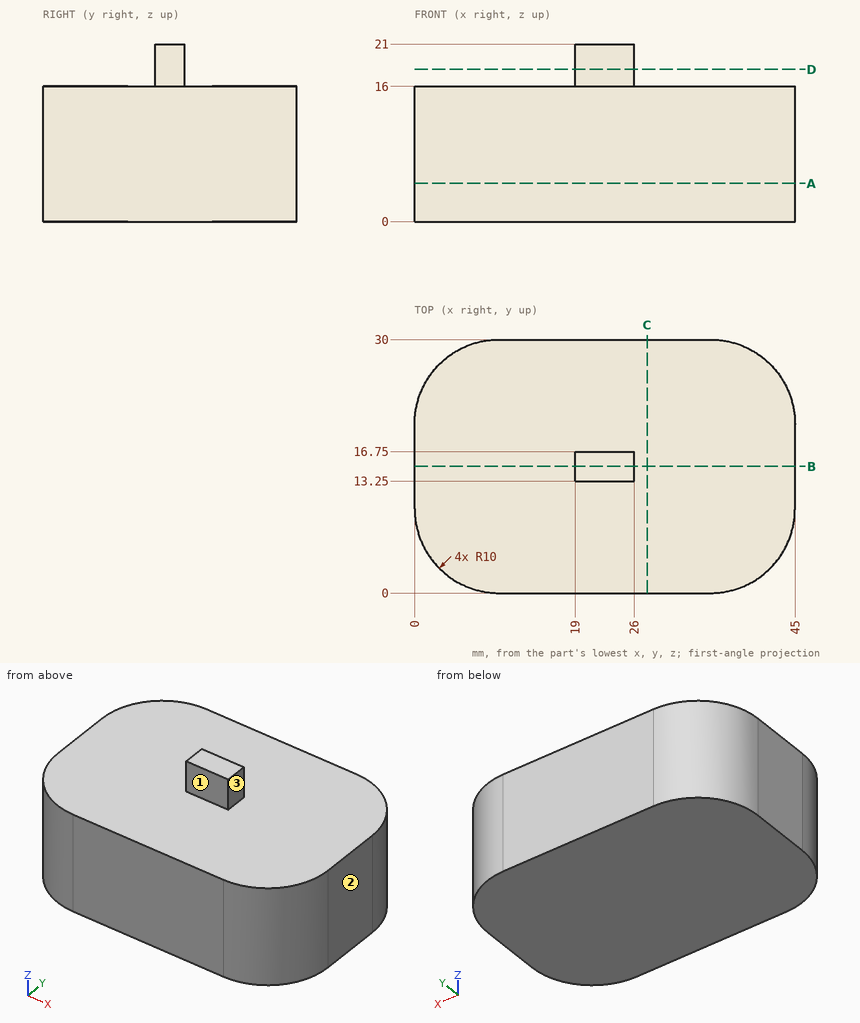
Here's the drawing with two shaded views (mm, measured from the low corner). I have some questions. A direction names the side the tool comes from. Coordinates: 2 decimals unless noted, no trailing zeros. Write each loop counter-clockwise with the first axis right and the second up, starting at its lowest first coordinate (ties: lowest second). Pieces come first, ordered by that corner, then holes. Notation, with made-up numbers: M -34.75,69 L 23.25,69 A22 cw 23.25,93 Z; hole C 14.25,-36.75 d9. An arc over 180 degrees is marked long. Answer as CSV lines item,"result".
Item 1: Imagine slicing it at B-B on y = 15. List the corners of the cut face in (x, z) for me, plus the area to 3 significant figures.
Geometry results:
outline,"M 0,0 L 45,0 L 45,16 L 26,16 L 26,21 L 19,21 L 19,16 L 0,16 Z"
area,"755 mm2"
Item 2: Imagine slicing it at A-A on z = 4.5. List the corners of the cut face in (x, y) for me.
Geometry results:
outline,"M 0,10 A10 ccw 10,0 L 35,0 A10 ccw 45,10 L 45,20 A10 ccw 35,30 L 10,30 A10 ccw 0,20 Z"
Item 3: I'm going to push flat-ended pins straight in: P1, Ø3, axis at y = 27, z = 9, coming from the +X side; P2, Ø1.5, axis at x = 24, z = 19.5, coming from the -Y side; P3, Ø2, axis at x = 7.5, y = 15, coming from the +Z side; P4, Ø6, axis at y = 7, z = 3, coming from the +X side. Where does each tip first touch, or does it pass through?
Geometry results:
P1,"stops at x = 43.35"
P2,"stops at y = 13.25"
P3,"stops at z = 16"
P4,"stops at x = 45"
Item 4: On a 3-axis mill with a long thin cutter (end or side, diameter ignored), from which of +Z, -Z, +X, -X, +Y, -Y can I reach the whole of each face in a straight line? I mean the marked faces 1, 2 and 3. Say none if no direction works.
Geometry results:
face 1,"+Z, +X, -X, -Y"
face 2,"+Z, -Z, +X, +Y, -Y"
face 3,"+Z, +X, +Y, -Y"
Item 5: Imagine slicing it at D-D on z = 18. List the corners of the cut face in (x, y) for me, plus the area to 3 significant figures.
Geometry results:
outline,"M 19,13.25 L 26,13.25 L 26,16.75 L 19,16.75 Z"
area,"24.5 mm2"
Item 6: Imagine slicing it at C-C on x = 27.5. List the corners of the cut face in (y, z) for me.
Geometry results:
outline,"M 0,0 L 30,0 L 30,16 L 0,16 Z"
Item 7: Please list where these lines run through material, in increasing order: line 1 along Z through (x, y) = (29.5, 19); line 2 along Y through (x, z) = (21, 19.5); line 3 along X through (y, z) = (8.5, 1.25).
Geometry results:
line 1,"z = 0 to 16"
line 2,"y = 13.25 to 16.75"
line 3,"x = 0.11 to 44.89"
